Can you work these out from the model? Positions are in its coordinate system, mm. A direction names the side the tool comes from. Round coordinates to 2 decimals unless told otherwise and drop trailing zeros. Loops run counter-clockwise (first coordinate to the right, second up) from the corner with the lowest first, then second, coordinate; pieces in that order, holes last. Notation, with made-up numbers: (-37, 38.25) -> (13, 38.25) arc R27 ccw to (13, 77.25) -> close; hole circle Ø8 at (-21, 60). An arc over 180 degrees is marked (long way). Answer as a JSON object with one key per item and string values.
```python
from build123d import *

# Parameters (mm, degrees)
ESBO_O1_R                = 1.75
RESSALTO_EXTRUS_O1_DEPTH = 5
ESBO_O4_W                = 30
ESBO_O4_H                = 20.000002677
RESSALTO_EXTRUS_O3_DEPTH = 5
ESBO_O5_R                = 3
CORTE_EXTRUS_O1_DEPTH    = 101.124923498
ESBO_O6_R                = 1.75
RESSALTO_EXTRUS_O5_DEPTH = 5
FILETE1_R                = 5
ESBO_O7_R                = 2
CORTE_EXTRUS_O2_DEPTH    = 101.124923498


with BuildPart() as part:
    # Esboço1 → Ressalto-extrusão1 (new body)
    with BuildSketch(Plane(origin=(0, 0, 0), x_dir=(1, 0, 0), z_dir=(0, 1, 0))):
        Polygon((-50, 0), (-50, 20.000002677), (-9.999996661, 60.000002546), (9.999996661, 60.000002546), (50, 20.000002677), (50, 0), align=None)
        with Locations(Location((-40, 10.000001339, 0), (0, 0, 270))):
            Circle(ESBO_O1_R, mode=Mode.SUBTRACT)
        with Locations(Location((-20, 10.000001339, 0), (0, 0, 270))):
            Circle(ESBO_O1_R, mode=Mode.SUBTRACT)
        with Locations(Location((0, 50.000002546, 0), (0, 0, 270))):
            Circle(ESBO_O1_R, mode=Mode.SUBTRACT)
        with Locations(Location((0, 30.000002546, 0), (0, 0, 270))):
            Circle(ESBO_O1_R, mode=Mode.SUBTRACT)
        with Locations(Location((20, 10.000001339, 0), (0, 0, 90))):
            Circle(ESBO_O1_R, mode=Mode.SUBTRACT)
        with Locations(Location((40, 10.000001339, 0), (0, 0, 90))):
            Circle(ESBO_O1_R, mode=Mode.SUBTRACT)
        with BuildLine():
            Line((-10, 43.443650782), (-10, 21.000001339))
            ThreePointArc((-10, 21.000001339), (-10.292893219, 20.292894558), (-11, 20.000001339))
            Line((-11, 20.000001339), (-33.443651391, 20.000001339))
            ThreePointArc((-33.443651391, 20.000001339), (-34.367530932, 20.617317926), (-34.150758141, 21.707108151))
            Line((-34.150758141, 21.707108151), (-11.707106751, 44.150757594))
            ThreePointArc((-11.707106751, 44.150757594), (-10.617316548, 44.367530307), (-10, 43.443650782))
        make_face(mode=Mode.SUBTRACT)
        with BuildLine():
            Line((11.707106751, 44.150757594), (34.150758141, 21.707108151))
            ThreePointArc((34.150758141, 21.707108151), (34.367530932, 20.617317926), (33.443651391, 20.000001339))
            Line((33.443651391, 20.000001339), (11, 20.000001339))
            ThreePointArc((11, 20.000001339), (10.292893219, 20.292894558), (10, 21.000001339))
            Line((10, 21.000001339), (10, 43.443650782))
            ThreePointArc((10, 43.443650782), (10.617316548, 44.367530307), (11.707106751, 44.150757594))
        make_face(mode=Mode.SUBTRACT)
    extrude(amount=RESSALTO_EXTRUS_O1_DEPTH)

    # Esboço4 → Ressalto-extrusão3 (add)
    with BuildSketch(Plane.XZ):
        with Locations((-65, -10.000001339)):
            Rectangle(ESBO_O4_W, ESBO_O4_H)
        with Locations((65, -10.000001339)):
            Rectangle(ESBO_O4_W, ESBO_O4_H)
    extrude(amount=-RESSALTO_EXTRUS_O3_DEPTH)

    # Esboço5 → Corte-extrusão1 (cut, through all)
    with BuildSketch(Plane.XZ):
        with Locations(Location((0, -40.000002546, 0), (0, 0, 270))):
            Circle(ESBO_O5_R)
    extrude(amount=-CORTE_EXTRUS_O1_DEPTH, mode=Mode.SUBTRACT)

    # Esboço6 → Ressalto-extrusão5 (add, through all)
    with BuildSketch(Plane.XZ):
        with Locations((0, -30.000002546)):
            Circle(ESBO_O6_R)
        with Locations((0, -50.000002546)):
            Circle(ESBO_O6_R)
    extrude(amount=-RESSALTO_EXTRUS_O5_DEPTH)

    # Filete1
    filete1_edges = [part.edges().sort_by_distance(p)[0] for p in [
        (-50, 2.5, -20.000002677),
        (-9.999996661, 2.5, -60.000002546),
        (9.999996661, 2.5, -60.000002546),
        (50, 2.5, -20.000002677),
        (-80, 2.5, -20.000002677),
        (-80, 2.5, 0),
        (80, 2.5, 0),
        (80, 2.5, -20.000002677),
    ]]
    fillet(filete1_edges, radius=FILETE1_R)

    # Esboço7 → Corte-extrusão2 (cut, through all)
    with BuildSketch(Plane.XZ):
        with Locations(Location((0, -50.000002546, 0), (0, 0, 270))):
            Circle(ESBO_O7_R)
        with Locations(Location((0, -30.000002546, 0), (0, 0, 270))):
            Circle(ESBO_O7_R)
    extrude(amount=-CORTE_EXTRUS_O2_DEPTH, mode=Mode.SUBTRACT)


solid = part.part
```
Q1. We'd pull the mould along Z, two halves only. Please class faces 1 (the flat face through (22, 2, -20)), 2 (the flat face through (-1, 5, -16)), 3 (the flat face through (63, 2, -20)): pulls with the +Z half, pulls with the -Z half, needs draft (parallel to the pull), parting line crosses it, or undercut.
Determined:
{"face 1": "undercut", "face 2": "needs draft", "face 3": "pulls with the -Z half"}
Q2. I want a section at A-A, the plane z = -50. Write out the boundary of the cut face in (x, y), then the cut area to 3 significant figures.
Determined:
{"outline": "(-20, 0) -> (-2, 0) -> (-2, 5) -> (-20, 5) -> close; (2, 0) -> (20, 0) -> (20, 5) -> (2, 5) -> close", "area": "180 mm²"}
Q3. I want a section at C-C, the plane x = -20. Write out the boundary of the cut face in (y, z).
Determined:
{"outline": "(0, -50) -> (5, -50) -> (5, -35.86) -> (0, -35.86) -> close; (0, -20) -> (5, -20) -> (5, -11.75) -> (0, -11.75) -> close; (0, -8.25) -> (5, -8.25) -> (5, 0) -> (0, 0) -> close"}
Q4. I'm going to push flat-ended pins straight in: pin 1 (2.5 mm diameter, centred on x = -66, y = 2.5, fed in from -Z); pin 2 (1.5 mm diameter, centred on y = 3, z = -32.5, fed in from +X). Where does each tip first touch, or does it pass through?
Determined:
{"pin 1": "z = -20", "pin 2": "x = 38.25"}
Q5. On a 3-axis mill with a long thin cutter (end or side, diameter ignored), from which of +Z, -Z, +X, -X, +Y, -Y can I reach the whole of each face in a straight line? I mean faces 4 (the flat face through (-10, 2, -32)), 5 (the flat face through (-64, 2, -20)), 6 (the cylindrical face through (50.13, 2.54, -20.39)). Say none if no direction works.
Determined:
{"face 4": "+Y, -Y", "face 5": "-Z, -X, +Y, -Y", "face 6": "-Z, +X, +Y, -Y"}
Q6. I want a section at B-B, the plane x = 40. Write out the boundary of the cut face in (y, z).
Determined:
{"outline": "(0, -30) -> (5, -30) -> (5, -11.75) -> (0, -11.75) -> close; (0, -8.25) -> (5, -8.25) -> (5, 0) -> (0, 0) -> close"}
Q7. I want a section at D-D, the plane z = -35. Write out the boundary of the cut face in (x, y), then the cut area to 3 significant figures.
Determined:
{"outline": "(-35, 0) -> (-20.86, 0) -> (-20.86, 5) -> (-35, 5) -> close; (-10, 0) -> (10, 0) -> (10, 5) -> (-10, 5) -> close; (20.86, 0) -> (35, 0) -> (35, 5) -> (20.86, 5) -> close", "area": "241 mm²"}
Q8. If I drill on L1, parallel to X at y = 3.6, z = -30; L2, parallel to Z at x = 58.5, y = 1.05; L3, parallel to X at y = 3.3, z = -35.5, over which ranges is the centre line in solid material (lowest first)? Write a range as [from, to].
Determined:
{"L1": "[-40, -25.86], [-10, -2], [2, 10], [25.86, 40]", "L2": "[-20, 0]", "L3": "[-34.5, -20.36], [-10, 10], [20.36, 34.5]"}
